Design review of the part built by this model. Coordinates are the model's own, in mm. A direction names the side the tool comes from. Coordinates: 2 decimals unless noted, no trailing zeros. Write each loop counter-clockwise with the first axis right and the second up, starting at its lowest first coordinate (ties: lowest second). Pieces come first, ordered by that corner, then holes. Notation, with made-up numbers: M 73.25,-39 L 106.25,-39 A18 ccw 106.25,-18 Z; hole C 2,19 d6. An arc over 180 degrees is marked long. One line per question, with ' | ' between items.
from build123d import *

# Parameters (mm, degrees)
SKETCH1_W           = 140
SKETCH1_H           = 140
BOSS_EXTRUDE1_DEPTH = 3
SKETCH2_W           = 16
SKETCH2_H           = 3
SKETCH2_W_2         = 3
SKETCH2_H_2         = 16
CUT_EXTRUDE1_DEPTH  = 3
SKETCH3_W           = 3
SKETCH3_H           = 10
CUT_EXTRUDE2_DEPTH  = 10
SKETCH4_W           = 3
SKETCH4_H           = 10
CUT_EXTRUDE3_DEPTH  = 3
CUT_EXTRUDE4_DEPTH  = 3
CUT_EXTRUDE5_DEPTH  = 3
BOSS_EXTRUDE4_DEPTH = 3
BOSS_EXTRUDE5_DEPTH = 3
SKETCH12_W          = 3
SKETCH12_H          = 3
BOSS_EXTRUDE6_DEPTH = 3
SKETCH13_W          = 3
SKETCH13_H          = 3
BOSS_EXTRUDE7_DEPTH = 3
BOSS_EXTRUDE8_DEPTH = 3
SKETCH15_W          = 140
SKETCH15_H          = 1
CUT_EXTRUDE6_DEPTH  = 3
SKETCH16_W          = 140
SKETCH16_H          = 70
CUT_EXTRUDE8_DEPTH  = 3
SKETCH17_R          = 3.99
CUT_EXTRUDE11_DEPTH = 3
SKETCH18_R          = 3.935
CUT_EXTRUDE12_DEPTH = 3


with BuildPart() as part:
    # Sketch1 → Boss-Extrude1 (new body)
    with BuildSketch(Plane(origin=(0, 0, 0), x_dir=(1, 0, 0), z_dir=(0, 1, 0))):
        Rectangle(SKETCH1_W, SKETCH1_H)
    extrude(amount=BOSS_EXTRUDE1_DEPTH)

    # Sketch2 → Cut-Extrude1 (cut)
    with BuildSketch(Plane(origin=(0, 3, 0), x_dir=(1, 0, 0), z_dir=(0, 1, 0))):
        with Locations((-22.5, 68.5)):
            Rectangle(SKETCH2_W, SKETCH2_H)
        with Locations((-22.5, -68.5)):
            Rectangle(SKETCH2_W, SKETCH2_H)
        with Locations((22.5, -68.5)):
            Rectangle(SKETCH2_W, SKETCH2_H)
        with Locations((22.5, 68.5)):
            Rectangle(SKETCH2_W, SKETCH2_H)
        with Locations((-68.5, 22.5)):
            Rectangle(SKETCH2_W_2, SKETCH2_H_2)
        with Locations((-68.5, -22.5)):
            Rectangle(SKETCH2_W_2, SKETCH2_H_2)
        with Locations((68.5, -22.5)):
            Rectangle(SKETCH2_W_2, SKETCH2_H_2)
        with Locations((68.5, 22.5)):
            Rectangle(SKETCH2_W_2, SKETCH2_H_2)
    extrude(amount=-CUT_EXTRUDE1_DEPTH, mode=Mode.SUBTRACT)

    # Sketch3 → Cut-Extrude2 (cut)
    with BuildSketch(Plane(origin=(0, 3, 0), x_dir=(1, 0, 0), z_dir=(0, 1, 0))):
        with Locations((-68.5, 65)):
            Rectangle(SKETCH3_W, SKETCH3_H)
    extrude(amount=-CUT_EXTRUDE2_DEPTH, mode=Mode.SUBTRACT)

    # Sketch4 → Cut-Extrude3 (cut)
    with BuildSketch(Plane(origin=(0, 3, 0), x_dir=(1, 0, 0), z_dir=(0, 1, 0))):
        with Locations((68.5, 65)):
            Rectangle(SKETCH4_W, SKETCH4_H)
    extrude(amount=-CUT_EXTRUDE3_DEPTH, mode=Mode.SUBTRACT)

    # Sketch5 → Cut-Extrude4 (cut)
    with BuildSketch(Plane(origin=(0, 3, 0), x_dir=(1, 0, 0), z_dir=(0, 1, 0))):
        Polygon((-21.03, 67), (-23.97, 67), (-23.97, 62.6), (-25.75, 62.6), (-25.75, 60), (-23.97, 60), (-23.97, 57.92), (-21.03, 57.92), (-21.03, 60), (-19.25, 60), (-19.25, 62.6), (-21.03, 62.6), align=None)
        Polygon((-21.03, -67), (-21.03, -62.6), (-19.25, -62.6), (-19.25, -60), (-21.03, -60), (-21.03, -57.92), (-23.97, -57.92), (-23.97, -60), (-25.75, -60), (-25.75, -62.6), (-23.97, -62.6), (-23.97, -67), align=None)
        Polygon((21.03, 67), (21.03, 62.6), (19.25, 62.6), (19.25, 60), (21.03, 60), (21.03, 57.92), (23.97, 57.92), (23.97, 60), (25.75, 60), (25.75, 62.6), (23.97, 62.6), (23.97, 67), align=None)
        Polygon((21.03, -67), (23.97, -67), (23.97, -62.6), (25.75, -62.6), (25.75, -60), (23.97, -60), (23.97, -57.92), (21.03, -57.92), (21.03, -60), (19.25, -60), (19.25, -62.6), (21.03, -62.6), align=None)
    extrude(amount=-CUT_EXTRUDE4_DEPTH, mode=Mode.SUBTRACT)

    # Sketch6 → Cut-Extrude5 (cut)
    with BuildSketch(Plane(origin=(0, 3, 0), x_dir=(1, 0, 0), z_dir=(0, 1, 0))):
        Polygon((67, -21.03), (67, -23.97), (62.6, -23.97), (62.6, -25.75), (60, -25.75), (60, -23.97), (57.92, -23.97), (57.92, -21.03), (60, -21.03), (60, -19.25), (62.6, -19.25), (62.6, -21.03), align=None)
        Polygon((67, 21.03), (62.6, 21.03), (62.6, 19.25), (60, 19.25), (60, 21.03), (57.92, 21.03), (57.92, 23.97), (60, 23.97), (60, 25.75), (62.6, 25.75), (62.6, 23.97), (67, 23.97), align=None)
        Polygon((-67, -21.03), (-62.6, -21.03), (-62.6, -19.25), (-60, -19.25), (-60, -21.03), (-57.92, -21.03), (-57.92, -23.97), (-60, -23.97), (-60, -25.75), (-62.6, -25.75), (-62.6, -23.97), (-67, -23.97), align=None)
        Polygon((-67, 21.03), (-67, 23.97), (-62.6, 23.97), (-62.6, 25.75), (-60, 25.75), (-60, 23.97), (-57.92, 23.97), (-57.92, 21.03), (-60, 21.03), (-60, 19.25), (-62.6, 19.25), (-62.6, 21.03), align=None)
    extrude(amount=-CUT_EXTRUDE5_DEPTH, mode=Mode.SUBTRACT)

    # Sketch8 → Boss-Extrude4 (add)
    with BuildSketch(Plane(origin=(0, 3, 0), x_dir=(1, 0, 0), z_dir=(0, 1, 0))):
        Polygon((-70, 30.5), (-67, 30.5), (-67, 23.97), (-62.6, 23.97), (-62.6, 25.75), (-60, 25.75), (-60, 23.97), (-57.92, 23.97), (-57.92, 21.03), (-60, 21.03), (-60, 19.25), (-62.6, 19.25), (-62.6, 21.03), (-67, 21.03), (-67, 14.5), (-70, 14.5), align=None)
    extrude(amount=-BOSS_EXTRUDE4_DEPTH)

    # Sketch10 → Boss-Extrude5 (add)
    with BuildSketch(Plane(origin=(0, 3, 0), x_dir=(1, 0, 0), z_dir=(0, 1, 0))):
        Polygon((70, 30.5), (67, 30.5), (67, 23.97), (62.6, 23.97), (62.6, 25.75), (60, 25.75), (60, 23.97), (57.92, 23.97), (57.92, 21.03), (60, 21.03), (60, 19.25), (62.6, 19.25), (62.6, 21.03), (67, 21.03), (67, 14.5), (70, 14.5), align=None)
    extrude(amount=-BOSS_EXTRUDE5_DEPTH)

    # Sketch12 → Boss-Extrude6 (add)
    with BuildSketch(Plane(origin=(0, 3, 0), x_dir=(1, 0, 0), z_dir=(0, 1, 0))):
        with Locations((-68.5, 68.5)):
            Rectangle(SKETCH12_W, SKETCH12_H)
    extrude(amount=-BOSS_EXTRUDE6_DEPTH)

    # Sketch13 → Boss-Extrude7 (add)
    with BuildSketch(Plane(origin=(0, 3, 0), x_dir=(1, 0, 0), z_dir=(0, 1, 0))):
        with Locations((68.5, 68.5)):
            Rectangle(SKETCH13_W, SKETCH13_H)
    extrude(amount=-BOSS_EXTRUDE7_DEPTH)

    # Sketch14 → Boss-Extrude8 (add)
    with BuildSketch(Plane(origin=(0, 3, 0), x_dir=(1, 0, 0), z_dir=(0, 1, 0))):
        Polygon((-30.5, 70), (-14.5, 70), (-14.5, 67), (-21.03, 67), (-21.03, 62.6), (-19.25, 62.6), (-19.25, 60), (-21.03, 60), (-21.03, 57.92), (-23.97, 57.92), (-23.97, 60), (-25.75, 60), (-25.75, 62.6), (-23.97, 62.6), (-23.97, 67), (-30.5, 67), align=None)
        Polygon((14.5, 70), (30.5, 70), (30.5, 67), (23.97, 67), (23.97, 62.6), (25.75, 62.6), (25.75, 60), (23.97, 60), (23.97, 57.92), (21.03, 57.92), (21.03, 60), (19.25, 60), (19.25, 62.6), (21.03, 62.6), (21.03, 67), (14.5, 67), align=None)
    extrude(amount=-BOSS_EXTRUDE8_DEPTH)

    # Sketch15 → Cut-Extrude6 (cut)
    with BuildSketch(Plane(origin=(0, 3, 0), x_dir=(1, 0, 0), z_dir=(0, 1, 0))):
        with Locations((0, -0.5)):
            Rectangle(SKETCH15_W, SKETCH15_H)
    extrude(amount=-CUT_EXTRUDE6_DEPTH, mode=Mode.SUBTRACT)

    # Sketch16 → Cut-Extrude8 (cut)
    with BuildSketch(Plane(origin=(0, 3, 0), x_dir=(1, 0, 0), z_dir=(0, 1, 0))):
        with Locations((0, 35)):
            Rectangle(SKETCH16_W, SKETCH16_H)
    extrude(amount=-CUT_EXTRUDE8_DEPTH, mode=Mode.SUBTRACT)

    # Sketch17 → Cut-Extrude11 (cut)
    with BuildSketch(Plane(origin=(0, 3, 0), x_dir=(1, 0, 0), z_dir=(0, 1, 0))):
        with Locations((0, -11)):
            Circle(SKETCH17_R)
        with Locations((-60, -60)):
            Circle(SKETCH17_R)
    extrude(amount=-CUT_EXTRUDE11_DEPTH, mode=Mode.SUBTRACT)

    # Sketch18 → Cut-Extrude12 (cut)
    with BuildSketch(Plane(origin=(0, 3, 0), x_dir=(1, 0, 0), z_dir=(0, 1, 0))):
        with Locations((-45, -59.9)):
            Circle(SKETCH18_R)
    extrude(amount=-CUT_EXTRUDE12_DEPTH, mode=Mode.SUBTRACT)


solid = part.part
1. Insertion check: pin 1 Ø9 at (x, z) = (0, 11) entering from -Y. The pin has a flat end and moves straight along its axis. Give the tip position at first contact, or say it passes through.
Answer sheet:
pin 1: y = 0
2. Tool access review of faces 1 (the face through (-69, 2, 14.5)), 2 (the face through (-19.25, 2, 61)), 3 (the face through (-51, 1, 70)), 4 (the face through (70, 2, 8)), 5 (the face through (18, 2, 67)): name each direction out of +Z, -Z, +X, -X, +Y, -Y from which nothing blocks a thin tool from reaching the whole face with its end or side.
Answer sheet:
face 1: -X, +Y, -Y | face 2: +Y, -Y | face 3: +Z, +X, -X, +Y, -Y | face 4: +Z, -Z, +X, +Y, -Y | face 5: +Z, +Y, -Y
3. Take a section at B-B (z = 11). Write out the cut boundary in (x, y), then the cut area to 3 significant figures.
Answer sheet:
outline: M -70,0 L -3.99,0 L -3.99,3 L -70,3 Z; M 3.99,0 L 70,0 L 70,3 L 3.99,3 Z | area: 396 mm^2
4. To check wall thickness, follow line 1 along X through (y, z) = (1.8, 59.9) (3 decimals); line 2 along X through (y, z) = (1.2, 11); line 3 along Z through (x, y) = (-45, 1.05) (3 decimals). State the ranges of each line that lie inside material, in increasing order. Write a range as [from, to].
Answer sheet:
line 1: [-70, -63.989], [-56.011, -48.935], [-41.065, -23.97], [-21.03, 21.03], [23.97, 70] | line 2: [-70, -3.99], [3.99, 70] | line 3: [1, 55.965], [63.835, 70]
5. Take a section at A-A (x = 0). Write out the cut boundary in (y, z).
Answer sheet:
outline: M 0,1 L 3,1 L 3,7.01 L 0,7.01 Z; M 0,14.99 L 3,14.99 L 3,70 L 0,70 Z
6. Take a section at C-C (y = 1.4). Count the separate pieces of the cut face and the enclosed holes in it, then the cut area to 3 significant figures.
Answer sheet:
separate pieces: 1 | enclosed holes: 3 | area: 9,180 mm^2
7. Draft analysis for pull direction X (two halves, no side actions). For faces 6 (the face through (65, 2, 21.03)), 7 (the face through (67, 2, 27)), 8 (the face through (19.25, 2, 61)), 9 (the face through (-61, 2, 19.25)), state which applies: pulls with the +X half, pulls with the -X half, needs draft (parallel to the pull), parting line crosses it, or undercut.
Answer sheet:
face 6: needs draft | face 7: pulls with the +X half | face 8: undercut | face 9: undercut
